Print and shaded views of the part. All mm, measured from the part's lowest x, y and z. A direction names the side the tool comes from. Coordinates: 2 decimals unless noted, no trailing zeros. Write each loop counter-clockwise with the first axis right and the second up, starting at its lowest first coordinate (ties: lowest second). Pieces come first, ordered by that corner, then holes. Notation, with made-up numbers: (9.25, 67) -> (29.25, 67) arc R17 ccw to (29.25, 90) -> close; hole circle Ø3 at (-32.5, -1.5). An arc over 180 degrees is marked (long way). Write item = value, one per line.
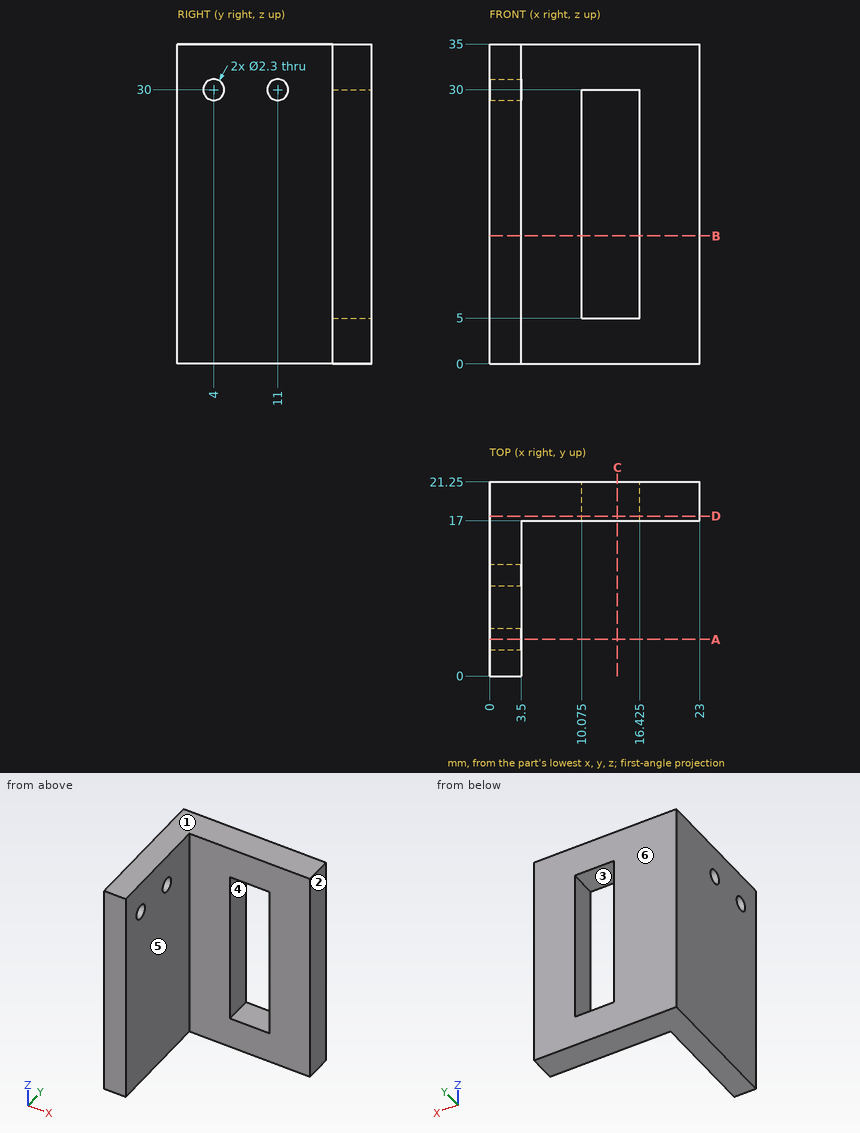
Q1. Probe line 1 (Z direction, x = 12, y = 18.5); line 2 (Z direction, x = 2.7, y = 4); line 3 (X direction, y = 19.25, z = 8) (3 decimals). List the from-to ranges inside material, lowest first. Write a range as from..to.
Model answer:
line_1 = 0..5, 30..35
line_2 = 0..28.85, 31.15..35
line_3 = 0..10.075, 16.425..23
Q2. Pin check, flat tips, straight feed: pin 1 (2 mm diameter, centred on y = 4, z = 30, fed in from -X); pin 2 (5 mm diameter, centred on x = 12.5, z = 25, fed in from -Y); pin 3 (10 mm diameter, centred on y = 11.5, z = 26.5, fed in from +X). Stop position of each tip, or through.
Model answer:
pin_1 = through
pin_2 = 17
pin_3 = 3.5
Q3. Saw through at D-D on y = 17.5. Give the cut face in (x, z) (3 decimals), and give its area (3 significant figures).
Model answer:
outline = (0, 0) -> (23, 0) -> (23, 35) -> (0, 35) -> close; hole (10.075, 5) -> (16.425, 5) -> (16.425, 30) -> (10.075, 30) -> close
area = 646 mm²
Q4. Saw through at A-A on y = 4. Give the cut face in (x, z).
Model answer:
outline = (0, 0) -> (3.5, 0) -> (3.5, 28.85) -> (0, 28.85) -> close; (0, 31.15) -> (3.5, 31.15) -> (3.5, 35) -> (0, 35) -> close
Q5. Saw through at B-B on z = 14. Give the cut face in (x, y) (3 decimals).
Model answer:
outline = (0, 0) -> (3.5, 0) -> (3.5, 17) -> (10.075, 17) -> (10.075, 21.25) -> (0, 21.25) -> close; (16.425, 17) -> (23, 17) -> (23, 21.25) -> (16.425, 21.25) -> close
Q6. Mould opens along Z. For the marked faces 1, 2 and 3 say: released by +Z, released by -Z, zero draft, split by the parting line, or undercut.
Model answer:
face_1 = released by +Z
face_2 = zero draft
face_3 = undercut
Q7. Which spindle directions (+Z, -Z, +X, -X, +Y, -Y) get a long thin tool onto all of the face, cutting with end or side? Do the marked faces 4, 5 and 6. Say none if no direction does.
Model answer:
face_4 = +Y, -Y
face_5 = +Z, -Z, +X, -Y
face_6 = +Z, -Z, +X, -X, +Y
Q8. Saw through at C-C on x = 14. Give the cut face in (y, z), and give its area (3 significant figures).
Model answer:
outline = (17, 0) -> (21.25, 0) -> (21.25, 5) -> (17, 5) -> close; (17, 30) -> (21.25, 30) -> (21.25, 35) -> (17, 35) -> close
area = 42.5 mm²
